```python
from build123d import *

# Parameters (mm, degrees)
SZKIC1_R                    = 63.5
DODANIE_WYCI_GNI_CIE2_DEPTH = 81.28
SZKIC2_R                    = 57.15
WYTNIJ_WYCI_GNI_CIE1_DEPTH  = 62.28
WYTNIJ_WYCI_GNI_CIE2_DEPTH  = 100
WYTNIJ_WYCI_GNI_CIE3_START  = -7.62
SZKIC5_R                    = 63.5
SZKIC5_R_2                  = 60.96
WYTNIJ_WYCI_GNI_CIE3_DEPTH  = 3.81
WYTNIJ_WYCI_GNI_CIE5_START  = -3.81
SZKIC6_R                    = 63.5
SZKIC6_R_2                  = 60.96
WYTNIJ_WYCI_GNI_CIE5_DEPTH  = 3.81
WYTNIJ_WYCI_GNI_CIE6_START  = 7.62
SZKIC7_R                    = 63.5
SZKIC7_R_2                  = 60.96
WYTNIJ_WYCI_GNI_CIE6_DEPTH  = 3.81
SZKIC8_W                    = 60.8
SZKIC8_H                    = 19
DODANIE_WYCI_GNI_CIE3_DEPTH = 63.5
SZKIC9_R                    = 12.7
WYTNIJ_WYCI_GNI_CIE7_DEPTH  = 144.237999261
ZAOKR_GLENIE3_R             = 10
ZAOKR_GLENIE4_R             = 5
ZAOKR_GLENIE5_R             = 5
WYTNIJ_WYCI_GNI_CIE8_START  = -1
SZKIC10_R                   = 13.2
SZKIC10_R_2                 = 12.7
WYTNIJ_WYCI_GNI_CIE8_DEPTH  = 1


with BuildPart() as part:
    # Szkic1 → Dodanie-wyciągnięcie2 (new body)
    with BuildSketch(Plane(origin=(0, 0, 0), x_dir=(1, 0, 0), z_dir=(0, 1, 0))):
        with Locations(Location((0, 0, 0), (0, 0, 270))):
            Circle(SZKIC1_R)
    extrude(amount=DODANIE_WYCI_GNI_CIE2_DEPTH)

    # Szkic2 → Wytnij-wyciągnięcie1 (cut)
    with BuildSketch(Plane(origin=(0, 81.28, 0), x_dir=(1, 0, 0), z_dir=(0, 1, 0))):
        with Locations(Location((0, 0, 0), (0, 0, 270))):
            Circle(SZKIC2_R)
    extrude(amount=-WYTNIJ_WYCI_GNI_CIE1_DEPTH, mode=Mode.SUBTRACT)

    # Szkic3 → Wytnij-wyciągnięcie2 (cut, symmetric)
    with BuildSketch(Plane.XY):
        with BuildLine():
            Line((-63.5, 81.28), (-63.5, 87.00412987))
            Line((-63.5, 87.00412987), (63.5, 87.00412987))
            Line((63.5, 87.00412987), (63.5, 81.28))
            Line((63.5, 81.28), (48.3, 81.28))
            ThreePointArc((48.3, 81.28), (41.228932188, 78.351067812), (38.3, 71.28))
            Line((38.3, 71.28), (38.3, 66.1))
            ThreePointArc((38.3, 66.1), (30.098989873, 46.301010127), (10.3, 38.1))
            Line((10.3, 38.1), (-10.3, 38.1))
            ThreePointArc((-10.3, 38.1), (-30.098989873, 46.301010127), (-38.3, 66.1))
            Line((-38.3, 66.1), (-38.3, 71.28))
            ThreePointArc((-38.3, 71.28), (-41.228932188, 78.351067812), (-48.3, 81.28))
            Line((-48.3, 81.28), (-63.5, 81.28))
        make_face()
    extrude(amount=WYTNIJ_WYCI_GNI_CIE2_DEPTH, both=True, mode=Mode.SUBTRACT)

    # Szkic5 → Wytnij-wyciągnięcie3 (cut)
    with BuildSketch(Plane(origin=(0, 0, 0), x_dir=(-1, 0, 0), z_dir=(0, -1, 0)).offset(WYTNIJ_WYCI_GNI_CIE3_START)):
        with Locations(Location((0, 0, 0), (0, 0, 90))):
            Circle(SZKIC5_R)
        with Locations(Location((0, 0, 0), (0, 0, 90))):
            Circle(SZKIC5_R_2, mode=Mode.SUBTRACT)
    extrude(amount=-WYTNIJ_WYCI_GNI_CIE3_DEPTH, mode=Mode.SUBTRACT)

    # Szkic6 → Wytnij-wyciągnięcie5 (cut)
    with BuildSketch(Plane(origin=(0, 11.43, 0), x_dir=(-1, 0, 0), z_dir=(0, -1, 0)).offset(WYTNIJ_WYCI_GNI_CIE5_START)):
        with Locations(Location((0, 0, 0), (0, 0, 90))):
            Circle(SZKIC6_R)
        with Locations(Location((0, 0, 0), (0, 0, 90))):
            Circle(SZKIC6_R_2, mode=Mode.SUBTRACT)
    extrude(amount=-WYTNIJ_WYCI_GNI_CIE5_DEPTH, mode=Mode.SUBTRACT)

    # Szkic7 → Wytnij-wyciągnięcie6 (cut)
    with BuildSketch(Plane(origin=(0, 15.24, 0), x_dir=(1, 0, 0), z_dir=(0, 1, 0)).offset(WYTNIJ_WYCI_GNI_CIE6_START)):
        with Locations(Location((0, 0, 0), (0, 0, 90))):
            Circle(SZKIC7_R)
        with Locations(Location((0, 0, 0), (0, 0, 90))):
            Circle(SZKIC7_R_2, mode=Mode.SUBTRACT)
    extrude(amount=WYTNIJ_WYCI_GNI_CIE6_DEPTH, mode=Mode.SUBTRACT)

    # Szkic8 → Dodanie-wyciągnięcie3 (add)
    with BuildSketch(Plane(origin=(0, 19, 0), x_dir=(1, 0, 0), z_dir=(0, 1, 0))):
        with Locations((0, 25.38)):
            Rectangle(SZKIC8_W, SZKIC8_H)
        with Locations((0, -25.38)):
            Rectangle(SZKIC8_W, SZKIC8_H)
    extrude(amount=DODANIE_WYCI_GNI_CIE3_DEPTH)

    # Szkic9 → Wytnij-wyciągnięcie7 (cut, through all)
    with BuildSketch(Plane.XY.offset(34.88)):
        with Locations((0, 57.1)):
            Circle(SZKIC9_R)
    extrude(amount=-WYTNIJ_WYCI_GNI_CIE7_DEPTH, mode=Mode.SUBTRACT)

    # Zaokrąglenie3
    zaokr_glenie3_edges = [part.edges().sort_by_distance(p)[0] for p in [
        (30.4, 82.5, -25.38),
        (-30.4, 82.5, -25.38),
        (30.4, 82.5, 25.38),
        (-30.4, 82.5, 25.38),
    ]]
    fillet(zaokr_glenie3_edges, radius=ZAOKR_GLENIE3_R)

    # Zaokrąglenie4
    zaokr_glenie4_edges = [part.edges().sort_by_distance(p)[0] for p in [
        (0, 82.5, -34.88),
        (0, 82.5, -15.88),
        (30.4, 45.75, -15.88),
        (-30.4, 45.75, -15.88),
        (27.471067812, 79.571067812, -15.88),
        (-27.471067812, 79.571067812, -15.88),
        (-30.4, 45.75, -34.88),
        (30.4, 45.75, -34.88),
        (27.471067812, 79.571067812, -34.88),
        (-27.471067812, 79.571067812, -34.88),
        (0, 82.5, 15.88),
        (0, 82.5, 34.88),
        (-30.4, 45.75, 15.88),
        (30.4, 45.75, 15.88),
        (-27.471067812, 79.571067812, 15.88),
        (27.471067812, 79.571067812, 15.88),
        (30.4, 45.75, 34.88),
        (-30.4, 45.75, 34.88),
        (-27.471067812, 79.571067812, 34.88),
        (27.471067812, 79.571067812, 34.88),
    ]]
    fillet(zaokr_glenie4_edges, radius=ZAOKR_GLENIE4_R)

    # Zaokrąglenie5
    zaokr_glenie5_edges = [part.edges().sort_by_distance(p)[0] for p in [
        (0, 19, -34.88),
        (30.4, 19, -25.38),
        (-30.4, 19, -25.38),
        (0, 19, -15.88),
        (0, 19, 34.88),
        (-30.4, 19, 25.38),
        (30.4, 19, 25.38),
        (0, 19, 15.88),
        (28.935533906, 19, -33.415533906),
        (-28.935533906, 19, -33.415533906),
        (-28.935533906, 19, -17.344466094),
        (28.935533906, 19, -17.344466094),
        (-28.935533906, 19, 33.415533906),
        (28.935533906, 19, 33.415533906),
        (28.935533906, 19, 17.344466094),
        (-28.935533906, 19, 17.344466094),
    ]]
    fillet(zaokr_glenie5_edges, radius=ZAOKR_GLENIE5_R)

    # Szkic10 → Wytnij-wyciągnięcie8 (cut)
    with BuildSketch(Plane.XY.offset(34.88).offset(WYTNIJ_WYCI_GNI_CIE8_START)):
        with Locations((0, 57.1)):
            Circle(SZKIC10_R)
        with Locations((0, 57.1)):
            Circle(SZKIC10_R_2, mode=Mode.SUBTRACT)
    wytnij_wyci_gni_cie8 = extrude(amount=-WYTNIJ_WYCI_GNI_CIE8_DEPTH, mode=Mode.SUBTRACT)

    # Lustro1: Wytnij-wyciągnięcie8 across plane
    add(wytnij_wyci_gni_cie8.mirror(Plane.XY), mode=Mode.SUBTRACT)


solid = part.part
```
Design review of the part built by this model. Coordinates are the model's own, in mm. A direction names the side the tool comes from. Coordinates: 2 decimals unless noted, no trailing zeros. Order: outer loops, then holes, each group sorted by start corner. A loop starts at its lowest first (then second) coordinate and runs counter-clockwise, first axis right, second up. Notation, with made-up numbers: (77.5, 16.5) -> (90.5, 16.5) arc R14 ccw to (90.5, 41.5) -> close; hole circle Ø4 at (33.5, 75). An arc over 180 degrees is marked (long way). One line per item, written item: value. Start each with the question number.
Q1. Take a section at A-A, the plane y = 35.5. State the section outline as (x, z) points.
Q2. Take a section at D-D, the plane x = 0. Give the number of separate pieces and of enclosed holes in the cut face, then the cut area to 3 significant figures.
Q3. Mouldability with a two-part tool opening along Z and no side actions: class faces 1 (the cylindrical face through (-61.99, 13.31, -13.77)), 2 (the cylindrical face through (-1.653, 69.692, -24.261)), 3 (the flat face through (-30.4, 48, 25)) as pulls with the +Z half, pulls with the -Z half, needs draft (parallel to the pull), parting line crosses it, or undercut.
Q4. For probe 1 along Z at (x, y) = (-20, 42); probe 2 along X at (y, z) = (57, 34); probe 3 along Z at (x, y) = (-30, 35.5), list the stretches that pass through material, from the lowest coordinate up.
Q5. Tool access review of faces 4 (the cylindrical face through (41.31, 78.43, -42.69)), 5 (the flat face through (-7, 68, 33.88)), 6 (the cylindrical face through (0.36, 20.43, 36.38)), 7 (the cylindrical face through (31.28, 47.56, 52.59)): name each direction out of +Z, -Z, +X, -X, +Y, -Y from which nothing blocks a thin tool from reaching the whole face with its end or side.
Q6. Insertion check: pin 1 Ø7 at (y, z) = (48.5, 25) entering from +X; pin 2 Ø4.5 at (x, z) = (-53.5, 0.5) entering from +Y; pin 3 Ø6 at (x, y) = (4.5, 26) entering from +Z. Each pin has a flat end and moves straight along its axis. Give the tip position at first contact, or say it passes through.
Values follow:
1. outline: circle Ø127 at (0, 0); (-30.4, -29.88) arc R5 ccw to (-25.4, -34.88) -> (25.4, -34.88) arc R5 ccw to (30.4, -29.88) -> (30.4, -20.88) arc R5 ccw to (25.4, -15.88) -> (-25.4, -15.88) arc R5 ccw to (-30.4, -20.88) -> close; (-30.4, 20.88) arc R5 ccw to (-25.4, 15.88) -> (25.4, 15.88) arc R5 ccw to (30.4, 20.88) -> (30.4, 29.88) arc R5 ccw to (25.4, 34.88) -> (-25.4, 34.88) arc R5 ccw to (-30.4, 29.88) -> close; hole circle Ø114.3 at (0, 0)
2. separate pieces: 3
2. enclosed holes: 0
2. area: 4,040 mm2
3. face 1: parting line crosses it
3. face 2: needs draft
3. face 3: undercut
4. probe 1: z = -34.88 to -15.88, 15.88 to 34.88
4. probe 2: x = -53.63 to -45.94, -28.23 to -12.7, 12.7 to 28.23, 45.94 to 53.63
4. probe 3: z = -55.97 to -48.64, -31.84 to -18.92, 18.92 to 31.84, 48.64 to 55.97
5. face 4: +Z, -Z, +Y
5. face 5: none
5. face 6: +Y
5. face 7: +Z, +Y
6. pin 1: stops at x = 59.75
6. pin 2: stops at y = 19
6. pin 3: stops at z = 63.48
